```python
from build123d import *

# Parameters (mm, degrees)
F0_W      = 40
F0_H      = 130
F1_DEPTH  = 250
F2_R      = 5
F3_DEPTH  = 15
F4_W      = 40
F4_H      = 130
F6_DEPTH  = 20
F5_R      = 5
F7_DEPTH  = 40
F8_R      = 5
F9_DEPTH  = 20
F10_DEPTH = 19.9


with BuildPart() as f1:
    # F0 (on Top) → F1 (new body)
    with BuildSketch(Plane.XY):
        with Locations((-20, -65)):
            Rectangle(F0_W, F0_H)
    extrude(amount=F1_DEPTH)

    # F2 (on face) → F3 (cut)
    with BuildSketch(Plane(origin=(0, 0, 0), x_dir=(-1, 0, 0), z_dir=(0, 1, 0))):
        with Locations((20, 150)):
            Circle(F2_R)
        with Locations((20, 100)):
            Circle(F2_R)
    extrude(amount=-F3_DEPTH, mode=Mode.SUBTRACT)

    # F4 (on face) → F6 (cut)
    with BuildSketch(Plane.XY.offset(250)):
        with Locations((-20, -65)):
            Rectangle(F4_W, F4_H)
    extrude(amount=-F6_DEPTH, mode=Mode.SUBTRACT)

    # F5 (on face) → F7 (cut)
    with BuildSketch(Plane.XY.offset(250)):
        with Locations((-20, -95)):
            Circle(F5_R)
    extrude(amount=-F7_DEPTH, mode=Mode.SUBTRACT)

    # F8 (on face) → F9 (cut)
    with BuildSketch(Plane(origin=(0, 0, 0), x_dir=(1, 0, 0), z_dir=(0, 0, -1))):
        with Locations((-20, 95)):
            Circle(F8_R)
    extrude(amount=-F9_DEPTH, mode=Mode.SUBTRACT)

    # F10 (add): a face of the model
    f10_faces = [f1.faces().sort_by_distance(p)[0] for p in [
        (-20, -64.53993697, 230),
    ]]
    extrude(f10_faces, amount=F10_DEPTH)


solid = f1.part
```
Part model, mm, in its own coordinate system. A direction names the side the tool comes from. Round coordinates to 2 decimals unless told otherwise and drop trailing zeros. Loops run counter-clockwise (first coordinate to the right, second up) from the corner with the lowest first, then second, coordinate; pieces in that order, holes last. Notation, with made-up numbers: (73.25, -40) -> (80.25, -40) arc R16 ccw to (80.25, -33) -> close; hole circle Ø11 at (-35, -14.5). An arc over 180 degrees is marked (long way). Use one line per item in the form item = value. Start each with the question number.
Item 1: Band-saw the part on D-D (z = 100). List the corners of the cut face in (x, y), plus the area to 3 significant figures.
Item 2: Drill centre lines: line 1 along Z through (x, y) = (-20, -6); line 2 along Y through (x, z) = (-20, 15); line 3 along X through (y, z) = (-95, 9). Where is each one in solid material? Low to high.
Item 3: Band-saw the part on B-B (z = 227.5). List the corners of the cut face in (x, y), plus the area to 3 significant figures.
Item 4: Band-saw the part on A-A (y = -95). List the corners of the cut face in (x, z).
Item 5: Drop a flat-ended pin along its axis: pin 1 Ø6 at (x, z) = (-20, 100) entering from +Y. Give the stop position or say it passes through.
Item 6: Two-plate mould, pull along X, no slides. Class faces 1 (the flat face through (-20, -15, 150)), 2 (the flat face through (0, -66, 123)), 3 (the flat face through (-20, 0, 123)), 4 (the cylindrical face through (-18.92, -7.4, 145.12)): released by +X, released by -X, zero draft, split by the parting line, or undercut.
Item 7: Band-saw the part on C-C (x = -20). List the corners of the cut face in (y, z), plus the area to 3 significant figures.
Item 8: Tool access for faces 5 (the flat face through (-20, -95, 210)), 6 (the cylindrical face through (-18.92, -7.4, 95.12)), 7 (the flat face through (-20, -95, 20)): list every direction of +Z, -Z, +X, -X, +Y, -Y with a clear straight run to the whole face (end or side of a thin tool).
Data:
q1.outline = (-40, -130) -> (0, -130) -> (0, 0) -> (-15, 0) -> (-15, -15) -> (-25, -15) -> (-25, 0) -> (-40, 0) -> close
q1.area = 5,050 mm^2
q2.line_1 = 0 to 95, 105 to 145, 155 to 249.9
q2.line_2 = -130 to -100, -90 to 0
q2.line_3 = -40 to -25, -15 to 0
q3.outline = (-40, -130) -> (0, -130) -> (0, 0) -> (-40, 0) -> close; hole circle Ø10 at (-20, -95)
q3.area = 5,120 mm^2
q4.outline = (-40, 0) -> (-25, 0) -> (-25, 20) -> (-15, 20) -> (-15, 0) -> (0, 0) -> (0, 249.9) -> (-15, 249.9) -> (-15, 210) -> (-25, 210) -> (-25, 249.9) -> (-40, 249.9) -> close
q5.pin_1 = -15
q6.face_1 = undercut
q6.face_2 = released by +X
q6.face_3 = zero draft
q6.face_4 = undercut
q7.outline = (-130, 0) -> (-100, 0) -> (-100, 20) -> (-90, 20) -> (-90, 0) -> (0, 0) -> (0, 95) -> (-15, 95) -> (-15, 105) -> (0, 105) -> (0, 145) -> (-15, 145) -> (-15, 155) -> (0, 155) -> (0, 249.9) -> (-90, 249.9) -> (-90, 210) -> (-100, 210) -> (-100, 249.9) -> (-130, 249.9) -> close
q7.area = 31,600 mm^2
q8.face_5 = +Z
q8.face_6 = +Y
q8.face_7 = -Z
